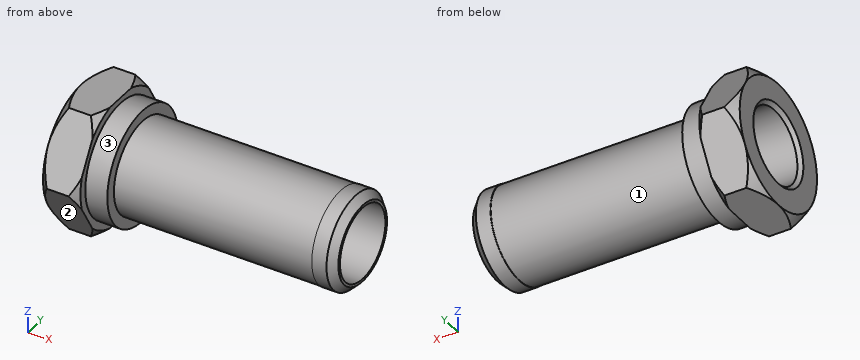
from build123d import *

# Parameters (mm, degrees)
SFAZOWANIE2_SIZE            = 1
SZKIC2_W                    = 27
SZKIC2_H                    = 0.05
SZKIC3_R                    = 5
DODANIE_WYCI_GNI_CIE1_DEPTH = 5.3
SFAZOWANIE3_SIZE            = 0.5


with BuildPart() as part:
    # Szkic1 → Obrót1 (revolve)
    with BuildSketch(Plane.XY, mode=Mode.PRIVATE) as obr_t1_sk:
        Polygon((0, 5), (33, 5), (33, 6.35), (3, 6.35), (3, 7.75), (0, 7.75), align=None)
    revolve(obr_t1_sk.sketch.rotate(Axis((0, 0, 0), (1, 0, 0)), 90), axis=Axis((0, 0, 0), (1, 0, 0)))

    # Sfazowanie2
    sfazowanie2_edges = [part.edges().sort_by_distance(p)[0] for p in [
        (33, 0, -6.35),
    ]]
    chamfer(sfazowanie2_edges, length=SFAZOWANIE2_SIZE)

    # Szkic2 → Wycięcie-obrót1 (revolve, cut)
    with BuildSketch(Plane.XY, mode=Mode.PRIVATE) as wyci_cie_obr_t1_sk:
        with Locations((16.5, 6.325)):
            Rectangle(SZKIC2_W, SZKIC2_H)
    revolve(wyci_cie_obr_t1_sk.sketch.rotate(Axis((3, 0, 0), (1, 0, 0)), 90), axis=Axis((3, 0, 0), (1, 0, 0)), mode=Mode.SUBTRACT)

    # Szkic3 → Dodanie-wyciągnięcie1 (add)
    with BuildSketch(Plane.ZY):
        Polygon((8.5, -4.907477288), (8.5, 4.907477288), (0, 9.814954576), (-8.5, 4.907477288), (-8.5, -4.907477288), (0, -9.814954576), align=None)
        Circle(SZKIC3_R, mode=Mode.SUBTRACT)
    extrude(amount=DODANIE_WYCI_GNI_CIE1_DEPTH)

    # Szkic4 → Wycięcie-obrót2 (revolve, cut)
    with BuildSketch(Plane(origin=(0, 0, 0), x_dir=(1, 0, 0), z_dir=(0, 1, 0)), mode=Mode.PRIVATE) as wyci_cie_obr_t2_sk:
        Polygon((-5.3, 8.5), (-5.3, 12), (-1.8, 12), align=None)
    revolve(wyci_cie_obr_t2_sk.sketch.rotate(Axis((0, 0, 0), (-1, 0, 0)), 180), axis=Axis((0, 0, 0), (-1, 0, 0)), mode=Mode.SUBTRACT)

    # Szkic5 → Wycięcie-obrót3 (revolve, cut)
    with BuildSketch(Plane.XY, mode=Mode.PRIVATE) as wyci_cie_obr_t3_sk:
        Polygon((0, -8.814954576), (0, -9.814954576), (-1, -9.814954576), align=None)
    revolve(wyci_cie_obr_t3_sk.sketch.rotate(Axis((0, 0, 0), (1, 0, 0)), 270), axis=Axis((0, 0, 0), (1, 0, 0)), mode=Mode.SUBTRACT)

    # Sfazowanie3
    sfazowanie3_edges = [part.edges().sort_by_distance(p)[0] for p in [
        (-5.3, 0, -5),
    ]]
    chamfer(sfazowanie3_edges, length=SFAZOWANIE3_SIZE)


solid = part.part
Part model, mm, in its own coordinate system. Face numbers are marked on the shaded views. A direction names the side the tool comes from. Coordinates: 2 decimals unless noted, no trailing zeros. Write each loop counter-clockwise with the first axis right and the second up, starting at its lowest first coordinate (ties: lowest second). Pieces come first, ordered by that corner, then holes. Notation, with made-up numbers: M -25.75,33.25 L -19.75,33.25 A9 cw -19.75,39.25 Z; hole C 39.25,66 d5. An arc over 180 degrees is marked long. Return JSON: item names as keys, results as strings.
1. Probe L1, parallel to Z at x = -2.85, y = 0; L2, parallel to Y at x = -1.9, z = 0; L3, parallel to Y at x = 13, z = -0.25. List the from-to ranges inside material, lowest first.
Determined:
{"L1": "-8.5 to -5, 5 to 8.5", "L2": "-9.81 to -5, 5 to 9.81", "L3": "-6.3 to -4.99, 4.99 to 6.3"}
2. 3-axis set-ups, long thin cutter, end or side, ignore diameter. For the marked faces 1, 2 and 3: which of +Z, -Z, +X, -X, +Y, -Y reach the whole face in a straight line?
Determined:
{"face 1": "none", "face 2": "-Z, +X, -X, -Y", "face 3": "+X"}
3. Saw through at A-A, the plane x = 27.5. Write the cut outline in (y, z).
Determined:
{"outline": "C 0,0 d12.6; hole C 0,0 d10"}
4. Flat gauge pins, fed straight in: pin 1 Ø1 at (x, z) = (9, 1.5) entering from +Y; pin 2 Ø1.5 at (x, z) = (1.5, -4) entering from +Y; pin 3 Ø10 at (y, z) = (0.5, 3) entering from -X; pin 4 Ø1.5 at (x, z) = (21, 5) entering from -Y. Where does each tip first touch, or does it go through?
Determined:
{"pin 1": "y = 6.22", "pin 2": "y = 7.04", "pin 3": "x = -5.3", "pin 4": "y = -4.65"}
